Input: dimensioned drawing with shaded views. Units: mm. Origin: part minimum x, y, z. Give positions to 0.01 mm unless a question says otherwise; leave off trailing zeros. Write each loop counter-clockwise with the first axis right and the second up, starting at its lowest first coordinate (ties: lowest second). Pieces come first, ordered by that corner, then holes. Notation, with made-up numbers: (26, 26.5) -> (74, 26.5) arc R23 cw to (74, 55.5) -> close; hole circle Ø1 at (3.25, -20.75). An arc over 180 degrees is marked (long way). Return JSON: item names as keys, results as strings. Group by question number.
Item 1: Section B-B, the plane x = 52. Return loops of the section in (y, z).
Item 2: Line query: line 1 (Z direction, x = 27, y = 57); line 2 (Y direction, x = 6.5, z = 95); line 3 (X direction, y = 26, z = 99.5) (1 decimal). Output: solid intervals per line, ascending. Write a range as [from, to].
Item 3: Pin query (flat end, axial travel): P1, Ø18, axis at x = 45, y = 40.5, coming from the +Z side; P2, Ø10.5, axis at x = 36.5, y = 52.5, coming from the -Z side; P3, Ø10, axis at x = 6, z = 99.5, coming from the -Y side. Return the tip coordinate at first contact, or that it passes through.
Item 4: Section A-A, the plane z = 98.5. Return loops of the section in (x, y) (1 decimal).
Item 5: Section C-C, the plane y = 7. Return loops of the section in (x, z), then the cut area to 3 significant figures.
Item 6: Section D-D, the plane z = 15.5. Return loops of the section in (x, y).
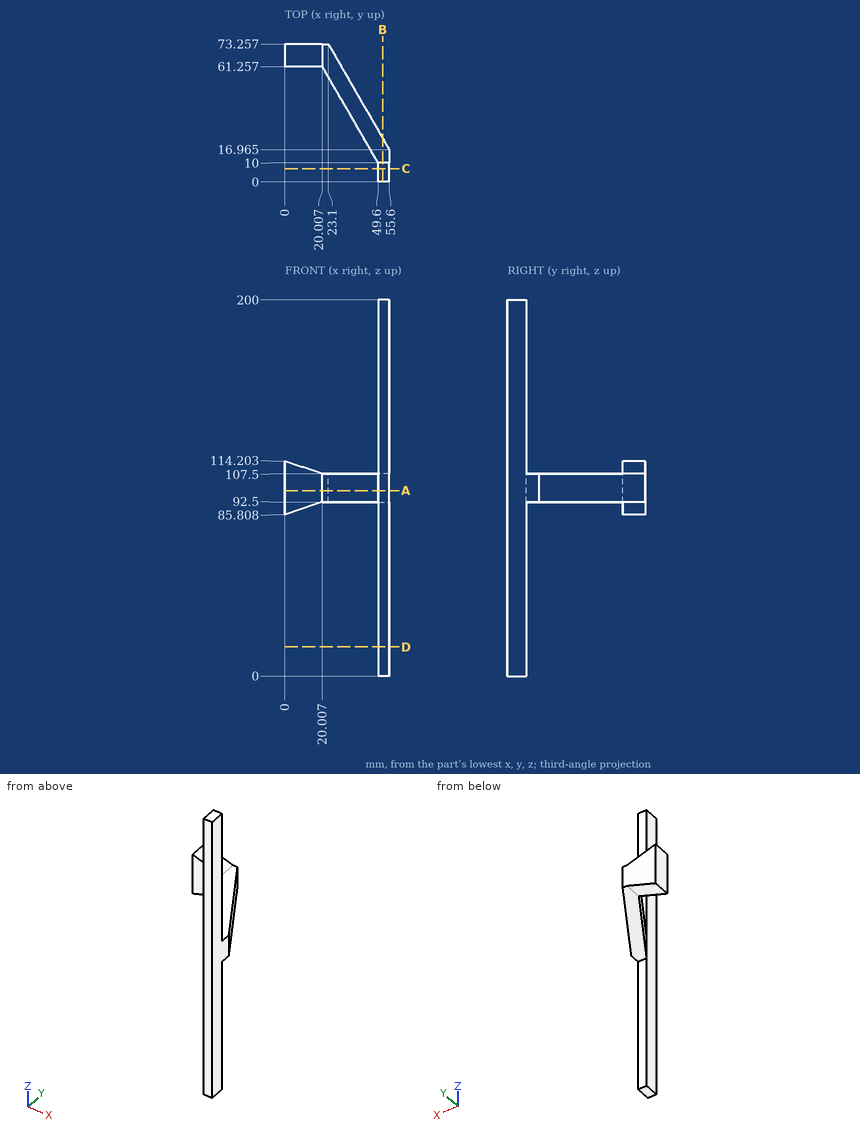
Answer below:
{
 "1": {"outline": "(0, 0) -> (10, 0) -> (10, 92.5) -> (23.2, 92.5) -> (23.2, 107.5) -> (10, 107.5) -> (10, 200) -> (0, 200) -> close"},
 "2": {"line 1": "z = [92.5, 107.5]", "line 2": "y = [61.26, 73.26]", "line 3": "x = [40.4, 50.4]"},
 "3": {"P1": "stops at z = 107.5", "P2": "stops at z = 92.5", "P3": "stops at y = 61.26"},
 "4": {"outline": "(0, 61.3) -> (20, 61.3) -> (49.6, 10) -> (49.6, 0) -> (55.6, 0) -> (55.6, 17) -> (23.1, 73.3) -> (0, 73.3) -> close"},
 "5": {"outline": "(49.6, 0) -> (55.6, 0) -> (55.6, 200) -> (49.6, 200) -> close", "area": "1,200 mm2"},
 "6": {"outline": "(49.6, 0) -> (55.6, 0) -> (55.6, 10) -> (49.6, 10) -> close"}
}
